Here's the drawing with two shaded views (mm, measured from the low corner). I have some questions. A direction names the side the tool comes from. Round coordinates to 2 decimals unless told otherwise and drop trailing zeros. Order: outer loops, then holes, each group sorted by start corner. A loop starts at its lowest first (then second) coordinate and runs counter-clockwise, first axis right, second up.
Q1. If we section it at D-D (x = 21): Please give me the cut outline in (y, z) (1 decimal).
Q2. Will these pins go through, and if not, where does the flat tip stop? P1, Ø2, axis at y = 52, z = 17.5, coming from the -X side; P2, Ø9.5, axis at x = 67, z = 8, coming from the +Y side; P3, Ø13.5, axis at x = 22, z = 17, coming from the +Y side.
Q3. For the marked faces 5, 6 and 7, which set-ups out of +Z, -Z, +X, -X, +Y, -Y let a thin tool reach every point of the face, with its end or its side?
Q4. If I drill on line 1 (Y direction, x = 66, z = 6.75) (1 decimal); line 2 (X direction, y = 37, z = 2.75) (1 decimal); line 3 (Y direction, x = 40, z = 25.25) (1 decimal), over which ranges is the centre line in solid material (lowest first)?
Q5. If we section it at C-C (y = 29): Please give me the cut outline in (x, z) (1 decimal).
Q6. If we section it at A-A (x = 48): Count the separate pieces of the cut face and the enclosed holes in it, plus the area to 3 significant figures.
Q7. We'd pull the mould along X, two halves only. Please class the marked faces 1, 2, 3 and 4: pulls with the +X half, pulls with the -X half, needs draft (parallel to the pull), parting line crosses it, or undercut.
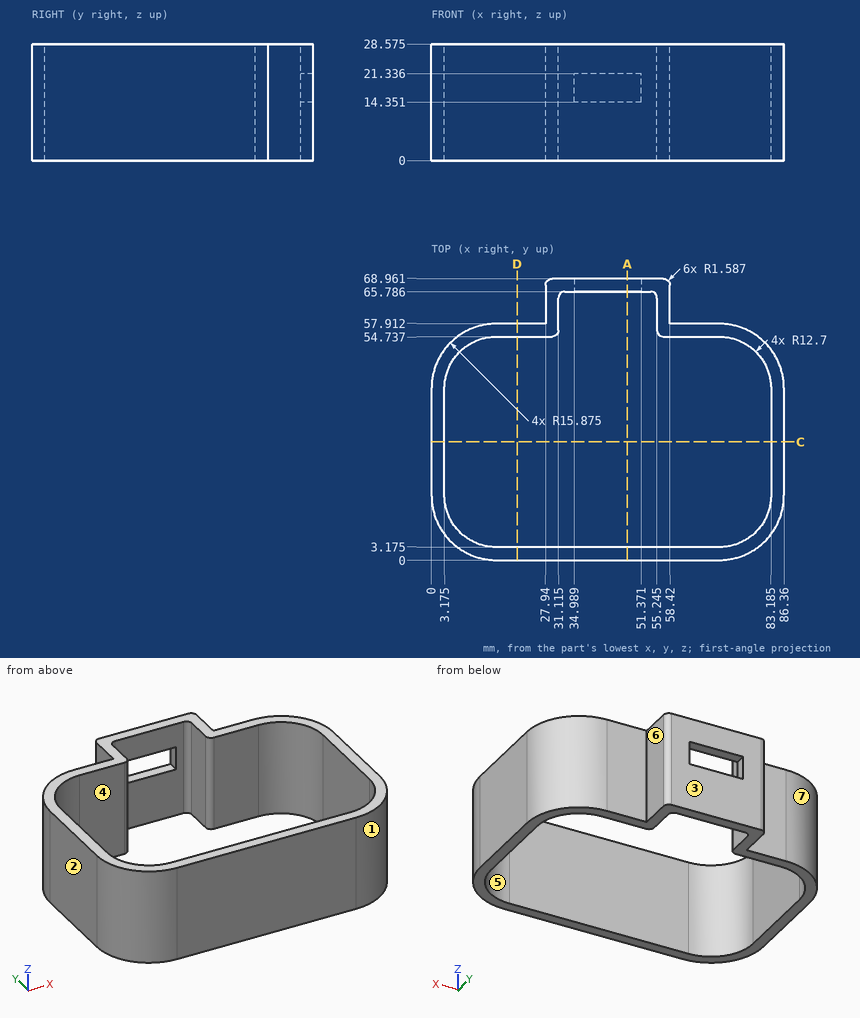
Solution:
1. outline: (0, 0) - (3.2, 0) - (3.2, 28.6) - (0, 28.6) - close; (54.7, 0) - (57.9, 0) - (57.9, 28.6) - (54.7, 28.6) - close
2. P1: stops at x = 2.77
2. P2: stops at y = 57.91
2. P3: stops at y = 68.76
3. face 5: +Z, -Z
3. face 6: +Z, -Z, +X, +Y
3. face 7: +Z, -Z, -X, +Y
4. line 1: y = 0 to 3.2, 54.7 to 57.9
4. line 2: x = 0 to 3.2, 83.2 to 86.4
4. line 3: y = 0 to 3.2, 65.8 to 69
5. outline: (0, 0) - (3.2, 0) - (3.2, 28.6) - (0, 28.6) - close; (83.2, 0) - (86.4, 0) - (86.4, 28.6) - (83.2, 28.6) - close
6. separate pieces: 3
6. enclosed holes: 0
6. area: 159 mm2
7. face 1: pulls with the +X half
7. face 2: pulls with the -X half
7. face 3: needs draft
7. face 4: undercut
